Here's how the part is built. I have some questions about the finished solid (model axes, mm). Round coordinates to 2 decimals unless told otherwise and drop trailing zeros. Loops run counter-clockwise (first coordinate to the right, second up) from the corner with the lowest first, then second, coordinate; pieces in that order, holes last. Notation, with made-up numbers: M 38.5,64 L 43.5,64 A28 cw 43.5,83 Z; hole C -3.5,46 d4. An arc over 180 degrees is marked long. Answer as CSV lines item,"result".
```python
from build123d import *

# Parameters (mm, degrees)
TUBO_CUADRADO_3_X_3_X_0_25_1_DEPTH = 1360
CROQUIS3_R                         = 6.35
CORTAR_EXTRUIR1_DEPTH              = 685.488860391
CROQUIS4_R                         = 6.35
CORTAR_EXTRUIR2_DEPTH              = 685.488860391


with BuildPart() as part:
    # Sketch1 → Tubo cuadrado 3 X 3 X 0.25(1) (new body)
    with BuildSketch(Plane(origin=(0, 0, -680), x_dir=(0, -1, 0), z_dir=(0, 0, 1))):
        with BuildLine():
            Line((-30, -35), (30, -35))
            ThreePointArc((30, -35), (33.535533906, -33.535533906), (35, -30))
            Line((35, -30), (35, 30))
            ThreePointArc((35, 30), (33.535533906, 33.535533906), (30, 35))
            Line((30, 35), (-30, 35))
            ThreePointArc((-30, 35), (-33.535533906, 33.535533906), (-35, 30))
            Line((-35, 30), (-35, -30))
            ThreePointArc((-35, -30), (-33.535533906, -33.535533906), (-30, -35))
        make_face()
        with BuildLine():
            Line((-30, -33), (30, -33))
            ThreePointArc((30, -33), (32.121320344, -32.121320344), (33, -30))
            Line((33, -30), (33, 30))
            ThreePointArc((33, 30), (32.121320344, 32.121320344), (30, 33))
            Line((30, 33), (-30, 33))
            ThreePointArc((-30, 33), (-32.121320344, 32.121320344), (-33, 30))
            Line((-33, 30), (-33, -30))
            ThreePointArc((-33, -30), (-32.121320344, -32.121320344), (-30, -33))
        make_face(mode=Mode.SUBTRACT)
    extrude(amount=TUBO_CUADRADO_3_X_3_X_0_25_1_DEPTH)

    # Croquis3 → Cortar-Extruir1 (cut, through all)
    with BuildSketch(Plane.XZ.offset(35)):
        with Locations(Location((0, 650, 0), (0, 0, 270))):
            Circle(CROQUIS3_R)
        with Locations(Location((0, 590, 0), (0, 0, 270))):
            Circle(CROQUIS3_R)
        with Locations(Location((0, -590, 0), (0, 0, 90))):
            Circle(CROQUIS3_R)
        with Locations(Location((0, -650, 0), (0, 0, 90))):
            Circle(CROQUIS3_R)
        with Locations(Location((0, -540, 0), (0, 0, 270))):
            Circle(CROQUIS3_R)
    extrude(amount=-CORTAR_EXTRUIR1_DEPTH, mode=Mode.SUBTRACT)

    # Croquis4 → Cortar-Extruir2 (cut, through all)
    with BuildSketch(Plane.ZY.offset(35)):
        with Locations((620, 0)):
            Circle(CROQUIS4_R)
    extrude(amount=-CORTAR_EXTRUIR2_DEPTH, mode=Mode.SUBTRACT)


solid = part.part
```
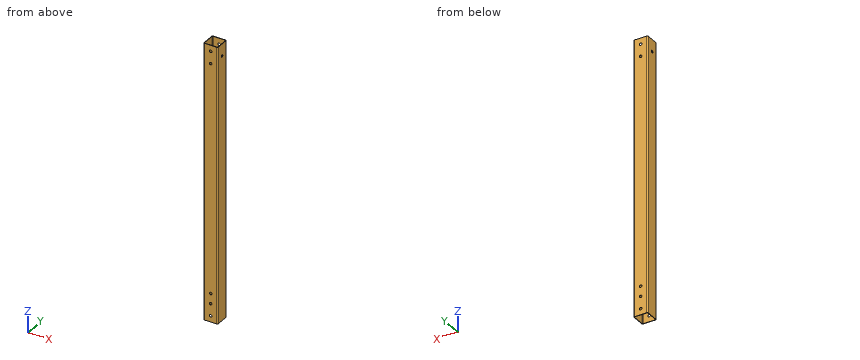
1. If I drill on line 1 (X direction, y = 34, z = -650); line 2 (Y direction, x = -14, z = 261), over which ranges is the centre line in solid material (lowest first)? Write a range as [from, to].
Evaluation:
line 1,"x = [-33, -6.35], [6.35, 33]"
line 2,"y = [-35, -33], [33, 35]"
2. I want a section at A-A, the plane z = -205. Please give me the cut outline in (x, y).
Evaluation:
outline,"M -35,-30 A5 ccw -30,-35 L 30,-35 A5 ccw 35,-30 L 35,30 A5 ccw 30,35 L -30,35 A5 ccw -35,30 Z; hole M -33,-30 A3 ccw -30,-33 L 30,-33 A3 ccw 33,-30 L 33,30 A3 ccw 30,33 L -30,33 A3 ccw -33,30 Z"
3. I want a section at B-B, the plane y = -18.5. Please give me the cut outline in (x, z).
Evaluation:
outline,"M -35,-680 L -33,-680 L -33,680 L -35,680 Z; M 33,-680 L 35,-680 L 35,680 L 33,680 Z"
